Part model, mm, in its own coordinate system. A direction names the side the tool comes from. Give positions to 0.01 mm unless a question says otherwise; leave off trailing zeros. Write each loop counter-clockwise with the first axis right and the second up, starting at its lowest first coordinate (ties: lowest second). Pieces come first, ordered by that corner, then holes.
```python
from build123d import *

# Parameters (mm, degrees)
SKETCH1_R           = 16
BOSS_EXTRUDE1_DEPTH = 12.5
SKETCH2_R           = 15
CUT_EXTRUDE1_DEPTH  = 10
SKETCH3_R           = 5
CUT_EXTRUDE2_DEPTH  = 10
SKETCH4_R           = 1
CUT_EXTRUDE3_DEPTH  = 10
SKETCH5_R           = 16
CUT_EXTRUDE4_DEPTH  = 0.5


with BuildPart() as part:
    # Sketch1 → Boss-Extrude1 (new body)
    with BuildSketch(Plane(origin=(0, 0, 0), x_dir=(1, 0, 0), z_dir=(0, 1, 0))):
        with Locations(Location((0, 0, 0), (0, 0, 270))):
            Circle(SKETCH1_R)
    extrude(amount=BOSS_EXTRUDE1_DEPTH)

    # Sketch2 → Cut-Extrude1 (cut)
    with BuildSketch(Plane(origin=(0, 12.5, 0), x_dir=(1, 0, 0), z_dir=(0, 1, 0))):
        with Locations(Location((0, 0, 0), (0, 0, 270))):
            Circle(SKETCH2_R)
    extrude(amount=-CUT_EXTRUDE1_DEPTH, mode=Mode.SUBTRACT)

    # Sketch3 → Cut-Extrude2 (cut)
    with BuildSketch(Plane(origin=(0, 0, 0), x_dir=(-1, 0, 0), z_dir=(0, -1, 0))):
        with Locations(Location((0, 0, 0), (0, 0, 90))):
            Circle(SKETCH3_R)
    extrude(amount=-CUT_EXTRUDE2_DEPTH, mode=Mode.SUBTRACT)

    # Sketch4 → Cut-Extrude3 (cut)
    with BuildSketch(Plane(origin=(0, 0, 0), x_dir=(-1, 0, 0), z_dir=(0, -1, 0))):
        with Locations(Location((0, 8, 0), (0, 0, 90))):
            Circle(SKETCH4_R)
        with Locations(Location((0, -8, 0), (0, 0, 90))):
            Circle(SKETCH4_R)
        with Locations(Location((-8, 0, 0), (0, 0, 90))):
            Circle(SKETCH4_R)
        with Locations(Location((8, 0, 0), (0, 0, 90))):
            Circle(SKETCH4_R)
    extrude(amount=-CUT_EXTRUDE3_DEPTH, mode=Mode.SUBTRACT)

    # Sketch5 → Cut-Extrude4 (cut)
    with BuildSketch(Plane.XZ):
        with Locations(Location((0, 0, 0), (0, 0, 270))):
            Circle(SKETCH5_R)
    extrude(amount=-CUT_EXTRUDE4_DEPTH, mode=Mode.SUBTRACT)


solid = part.part
```
1) Saw through at C-C, the plane x = -8. Write the cut outline in (y, z), then the cut area to 3 significant figures.
Answers follow:
outline: (0.5, -13.86) - (12.5, -13.86) - (12.5, -12.69) - (2.5, -12.69) - (2.5, -1) - (0.5, -1) - close; (0.5, 1) - (2.5, 1) - (2.5, 12.69) - (12.5, 12.69) - (12.5, 13.86) - (0.5, 13.86) - close
area: 74.8 mm2
2) Saw through at D-D, the plane y = 1.75. Write the cut outline in (x, z).
Answers follow:
outline: circle Ø32 at (0, 0); hole circle Ø2 at (-8, 0); hole circle Ø10 at (0, 0); hole circle Ø2 at (0, -8); hole circle Ø2 at (0, 8); hole circle Ø2 at (8, 0)
3) Two-plate mould, pull along X, no slides. Class faces 1 (the face through (-15.62, 6.42, -3.47)), 2 (the face through (4, 0.5, 4)), 3 (the face through (4, 2.5, -4)): +X half, -X half, draft (parallel to the pull), parting line (faces both ways), or undercut.
Answers follow:
face 1: parting line
face 2: draft
face 3: undercut
4) Saw through at A-A, the plane x = 0. Write the cut outline in (y, z).
Answers follow:
outline: (0.5, -16) - (12.5, -16) - (12.5, -15) - (2.5, -15) - (2.5, -9) - (0.5, -9) - close; (0.5, -7) - (2.5, -7) - (2.5, -5) - (0.5, -5) - close; (0.5, 5) - (2.5, 5) - (2.5, 7) - (0.5, 7) - close; (0.5, 9) - (2.5, 9) - (2.5, 15) - (12.5, 15) - (12.5, 16) - (0.5, 16) - close
5) Saw through at B-B, the plane z = 0. Write the cut outline in (x, y).
Answers follow:
outline: (-16, 0.5) - (-9, 0.5) - (-9, 2.5) - (-15, 2.5) - (-15, 12.5) - (-16, 12.5) - close; (-7, 0.5) - (-5, 0.5) - (-5, 2.5) - (-7, 2.5) - close; (5, 0.5) - (7, 0.5) - (7, 2.5) - (5, 2.5) - close; (9, 0.5) - (16, 0.5) - (16, 12.5) - (15, 12.5) - (15, 2.5) - (9, 2.5) - close
6) 3-axis set-ups, long thin cutter, end or side, ignore diameter. For faces 4 (the face through (-0.6, 1.5, 8.8)), 5 (the face through (0.66, 7.57, -14.985)): which of +Z, -Z, +X, -X, +Y, -Y reach the whole face in a straight line?
Answers follow:
face 4: +Y, -Y
face 5: +Y
7) Wall check: L1, parallel to X at y = 1.4, z = 0; L2, parallel to X at y = 10.5, z = 0.5; L3, parallel to Y at x = 9.5, z = -1. Give the ranges that are in metal, low to high.
Answers follow:
L1: x = -16 to -9, -7 to -5, 5 to 7, 9 to 16
L2: x = -15.99 to -14.99, 14.99 to 15.99
L3: y = 0.5 to 2.5
8) Pin check, flat tips, straight feed: pin 1 Ø13 at (x, z) = (0, 0) entering from +Y; pin 2 Ø2 at (x, y) = (-12.5, 9.5) entering from +Z; pin 3 Ø1 at (y, z) = (10.5, -4.5) entering from -X; pin 4 Ø1.6 at (x, z) = (0, 8) entering from +Y (3 decimals). Stop position of each tip, or through.
Answers follow:
pin 1: stops at y = 2.5
pin 2: stops at z = 11.12
pin 3: stops at x = -15.49
pin 4: passes through
